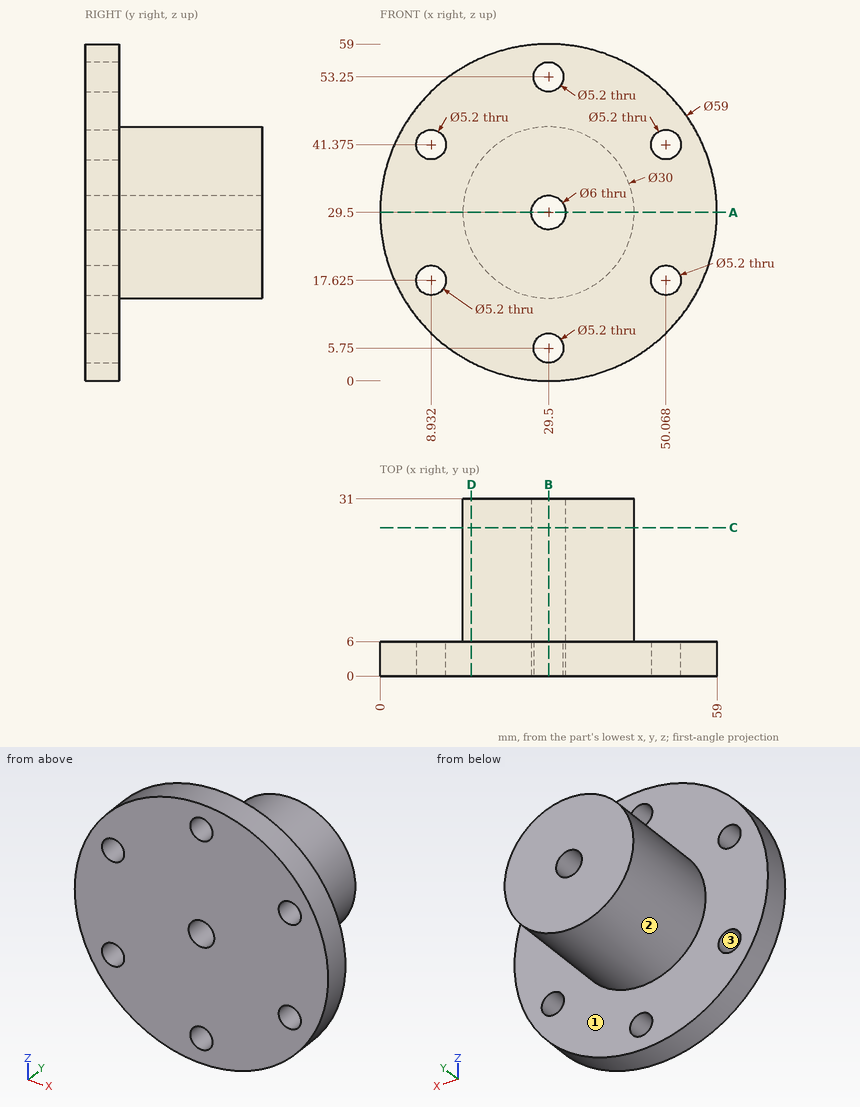
Geometry check sheet. Reference: drawing and pictorial views, mm from the part's lowest x, y, z. Coordinates: 2 decimals unless noted, no trailing zeros. Write each loop counter-clockwise with the first axis right and the second up, starting at its lowest first coordinate (ties: lowest second). Pieces come first, ordered by that corner, then holes. Notation, with made-up numbers: (23, -36.75) - (27, -36.75) arc R23 ccw to (27, -10.75) - close; hole circle Ø5 at (46.5, -13.5). An arc over 180 degrees is marked (long way). Write item = value, one per line.
Q1. Mould release check, pull along Z, two halves, no side actions. Record for the marked faces 1, 2 and 3: released by +Z, released by -Z, zero draft, split by the parting line, or undercut.
Answer:
face_1 = zero draft
face_2 = split by the parting line
face_3 = undercut
Q2. Material ranges on L1, parallel to Z at x = 29.5, y = 2.9; L2, parallel to Z at x = 29.5, y = 25.5; L3, parallel to Y at x = 8.5, z = 26, recorded low to high. Write a range as from..to.
Answer:
L1 = 0..3.15, 8.35..26.5, 32.5..50.65, 55.85..59
L2 = 14.5..26.5, 32.5..44.5
L3 = 0..6
Q3. Cross-section at D-D (x = 16). Enter the section's corners in (y, z), plus the area to 3 significant figures.
Answer:
outline = (0, 3.27) - (6, 3.27) - (6, 22.96) - (31, 22.96) - (31, 36.04) - (6, 36.04) - (6, 55.73) - (0, 55.73) - close
area = 642 mm²
Q4. Go/stop test with flat-tipped pins: pin 1 Ø8 at (x, z) = (20, 50) entering from +Y; pin 2 Ø4 at (y, z) = (7.5, 12.5) entering from -X; pin 3 Ø2 at (x, y) = (15.5, 5.5) entering from +Z. Record where each tip stops, or that it passes through.
Answer:
pin_1 = 6
pin_2 = 4.51
pin_3 = 55.98
Q5. Cross-section at A-A (z = 29.5). Enter the section's corners in (x, y), plus the area to 3 significant figures.
Answer:
outline = (0, 0) - (26.5, 0) - (26.5, 31) - (14.5, 31) - (14.5, 6) - (0, 6) - close; (32.5, 0) - (59, 0) - (59, 6) - (44.5, 6) - (44.5, 31) - (32.5, 31) - close
area = 918 mm²
Q6. Cross-section at B-B (x = 29.5). Enter the section's corners in (y, z).
Answer:
outline = (0, 0) - (6, 0) - (6, 3.15) - (0, 3.15) - close; (0, 8.35) - (6, 8.35) - (6, 14.5) - (31, 14.5) - (31, 26.5) - (0, 26.5) - close; (0, 32.5) - (31, 32.5) - (31, 44.5) - (6, 44.5) - (6, 50.65) - (0, 50.65) - close; (0, 55.85) - (6, 55.85) - (6, 59) - (0, 59) - close
Q7. Cross-section at C-C (y = 26). Enter the section's corners in (x, z).
Answer:
outline = circle Ø30 at (29.5, 29.5); hole circle Ø6 at (29.5, 29.5)
